```python
from build123d import *

# Parameters (mm, degrees)
SKETCH_1_W             = 800
SKETCH_1_H             = 400
EXTRUDE_1_DEPTH        = 20
SKETCH_3_W             = 302
SKETCH_3_H             = 352
CUT_EXTRUDE_1_DEPTH    = 5
CUT_EXTRUDE_2_DEPTH    = 2.7
FILLET_1_R             = 0.13
FILLET_2_R             = 0.5
FILLET_3_R             = 10
CUT_EXTRUDE_3_DEPTH    = 448.465082437
SKETCH_10_R            = 5.5
SKETCH_10_R_2          = 5
CUT_EXTRUDE_4_DEPTH    = 7
SKETCH_11_R            = 3.25
CUT_EXTRUDE_5_DEPTH    = 448.660585712
HOLE_WIZARD_M5_2_D     = 4.2
HOLE_WIZARD_M5_2_DEPTH = 14
HOLE_WIZARD_M5_2_TIP   = 1.2618073


with BuildPart() as part:
    # 스케치1 → 보스-돌출1 (new body)
    with BuildSketch(Plane(origin=(0, 0, 0), x_dir=(1, 0, 0), z_dir=(0, 1, 0))):
        Rectangle(SKETCH_1_W, SKETCH_1_H)
    extrude(amount=EXTRUDE_1_DEPTH)

    # 스케치3 → 컷-돌출1 (cut)
    with BuildSketch(Plane(origin=(0, 20, 0), x_dir=(1, 0, 0), z_dir=(0, 1, 0))):
        with Locations((200, 0)):
            Rectangle(SKETCH_3_W, SKETCH_3_H)
    extrude(amount=-CUT_EXTRUDE_1_DEPTH, mode=Mode.SUBTRACT)

    # 스케치4 → 컷-돌출2 (cut)
    with BuildSketch(Plane(origin=(0, 15, 0), x_dir=(1, 0, 0), z_dir=(0, 1, 0))):
        with BuildLine():
            Line((73.5, 168.55), (326.5, 168.55))
            ThreePointArc((326.5, 168.55), (338.556170619, 163.556170619), (343.55, 151.5))
            Line((343.55, 151.5), (343.55, -151.5))
            ThreePointArc((343.55, -151.5), (338.556170619, -163.556170619), (326.5, -168.55))
            Line((326.5, -168.55), (73.5, -168.55))
            ThreePointArc((73.5, -168.55), (61.443829381, -163.556170619), (56.45, -151.5))
            Line((56.45, -151.5), (56.45, 151.5))
            ThreePointArc((56.45, 151.5), (61.443829381, 163.556170619), (73.5, 168.55))
        make_face()
        with BuildLine():
            Line((73.5, 164.45), (326.5, 164.45))
            ThreePointArc((326.5, 164.45), (335.657032816, 160.657032816), (339.45, 151.5))
            Line((339.45, 151.5), (339.45, -151.5))
            ThreePointArc((339.45, -151.5), (335.657032816, -160.657032816), (326.5, -164.45))
            Line((326.5, -164.45), (73.5, -164.45))
            ThreePointArc((73.5, -164.45), (64.342967184, -160.657032816), (60.55, -151.5))
            Line((60.55, -151.5), (60.55, 151.5))
            ThreePointArc((60.55, 151.5), (64.342967184, 160.657032816), (73.5, 164.45))
        make_face(mode=Mode.SUBTRACT)
    extrude(amount=-CUT_EXTRUDE_2_DEPTH, mode=Mode.SUBTRACT)

    # 필렛1
    fillet_1_edges = [part.edges().sort_by_distance(p)[0] for p in [
        (61.443829381, 15, -163.556170619),
        (56.45, 15, 0),
        (61.443829381, 15, 163.556170619),
        (200, 15, 168.55),
        (338.556170619, 15, 163.556170619),
        (343.55, 15, 0),
        (338.556170619, 15, -163.556170619),
        (200, 15, -168.55),
        (64.342967184, 15, -160.657032816),
        (200, 15, -164.45),
        (335.657032816, 15, -160.657032816),
        (339.45, 15, 0),
        (335.657032816, 15, 160.657032816),
        (200, 15, 164.45),
        (64.342967184, 15, 160.657032816),
        (60.55, 15, 0),
    ]]
    fillet(fillet_1_edges, radius=FILLET_1_R)

    # 필렛2
    fillet_2_edges = [part.edges().sort_by_distance(p)[0] for p in [
        (61.443829381, 12.3, -163.556170619),
        (200, 12.3, -168.55),
        (338.556170619, 12.3, -163.556170619),
        (343.55, 12.3, 0),
        (338.556170619, 12.3, 163.556170619),
        (200, 12.3, 168.55),
        (61.443829381, 12.3, 163.556170619),
        (56.45, 12.3, 0),
        (200, 12.3, -164.45),
        (64.342967184, 12.3, -160.657032816),
        (60.55, 12.3, 0),
        (64.342967184, 12.3, 160.657032816),
        (200, 12.3, 164.45),
        (335.657032816, 12.3, 160.657032816),
        (339.45, 12.3, 0),
        (335.657032816, 12.3, -160.657032816),
    ]]
    fillet(fillet_2_edges, radius=FILLET_2_R)

    # 필렛3
    fillet_3_edges = [part.edges().sort_by_distance(p)[0] for p in [
        (351, 17.5, -176),
        (351, 17.5, 176),
        (49, 17.5, 176),
        (49, 17.5, -176),
    ]]
    fillet(fillet_3_edges, radius=FILLET_3_R)

    # 스케치6 → 컷-돌출3 (cut, through all)
    with BuildSketch(Plane(origin=(0, 15, 0), x_dir=(1, 0, 0), z_dir=(0, 1, 0))):
        with BuildLine():
            Line((80, 155), (320, 155))
            ThreePointArc((320, 155), (327.071067812, 152.071067812), (330, 145))
            Line((330, 145), (330, -145))
            ThreePointArc((330, -145), (327.071067812, -152.071067812), (320, -155))
            Line((320, -155), (80, -155))
            ThreePointArc((80, -155), (72.928932188, -152.071067812), (70, -145))
            Line((70, -145), (70, 145))
            ThreePointArc((70, 145), (72.928932188, 152.071067812), (80, 155))
        make_face()
    extrude(amount=-CUT_EXTRUDE_3_DEPTH, mode=Mode.SUBTRACT)

    # 스케치10 → 컷-돌출4 (cut)
    with BuildSketch(Plane(origin=(0, 20, 0), x_dir=(1, 0, 0), z_dir=(0, 1, 0))):
        with Locations(Location((0, 190, 0), (0, 0, 270))):
            Circle(SKETCH_10_R)
        with Locations(Location((-390, 190, 0), (0, 0, 270))):
            Circle(SKETCH_10_R)
        with Locations(Location((-390, -190, 0), (0, 0, 270))):
            Circle(SKETCH_10_R)
        with Locations(Location((0, -190, 0), (0, 0, 270))):
            Circle(SKETCH_10_R)
        with Locations(Location((390, -190, 0), (0, 0, 270))):
            Circle(SKETCH_10_R_2)
        with Locations(Location((390, 190, 0), (0, 0, 270))):
            Circle(SKETCH_10_R_2)
    extrude(amount=-CUT_EXTRUDE_4_DEPTH, mode=Mode.SUBTRACT)

    # 스케치11 → 컷-돌출5 (cut, through all)
    with BuildSketch(Plane(origin=(0, 20, 0), x_dir=(1, 0, 0), z_dir=(0, 1, 0))):
        with Locations(Location((-390, 190, 0), (0, 0, 270))):
            Circle(SKETCH_11_R)
        with Locations(Location((0, 190, 0), (0, 0, 270))):
            Circle(SKETCH_11_R)
        with Locations(Location((0, -190, 0), (0, 0, 270))):
            Circle(SKETCH_11_R)
        with Locations(Location((-390, -190, 0), (0, 0, 270))):
            Circle(SKETCH_11_R)
        with Locations(Location((390, -190, 0), (0, 0, 270))):
            Circle(SKETCH_11_R)
        with Locations(Location((390, 190, 0), (0, 0, 270))):
            Circle(SKETCH_11_R)
    extrude(amount=-CUT_EXTRUDE_5_DEPTH, mode=Mode.SUBTRACT)

    # M5 나사 구멍2
    with Locations(Plane(origin=(0, 20, 0), x_dir=(1, 0, 0), z_dir=(0, 1, 0))):
        with Locations((8.5, 120.5), (38.5, 120.5), (8.5, 60.5), (38.5, 60.5), (8.5, -60.5), (38.5, -60.5), (8.5, -120.5), (38.5, -120.5)):
            Hole(HOLE_WIZARD_M5_2_D / 2, depth=HOLE_WIZARD_M5_2_DEPTH)
            with Locations((0, 0, -(HOLE_WIZARD_M5_2_DEPTH + HOLE_WIZARD_M5_2_TIP / 2))):  # 118° drill point
                Cone(0, HOLE_WIZARD_M5_2_D / 2, HOLE_WIZARD_M5_2_TIP, mode=Mode.SUBTRACT)


solid = part.part
```
The listing builds one solid part. Answer for the finished solid, in the listing's coordinates (mm). A direction names the side the tool comes from. Give positions to 0.01 mm unless a question says otherwise; leave off trailing zeros. Order: outer loops, then holes, each group sorted by start corner. A loop starts at its lowest first (then second) coordinate and runs counter-clockwise, first axis right, second up. Notation, with made-up numbers: (15, 89.5) -> (20, 89.5) arc R21 cw to (20, 124.5) -> close; hole circle Ø2 at (67.5, 81). An arc over 180 degrees is marked (long way). Answer as a JSON object with one key per item and string values. Group by question number.
Item 1: A tool of negligible diameter and unlimited length cuts with its end or side. For faces 5 (the flat face through (-183, 20, -3)), 6 (the flat face through (202, 8, 155)), 7 (the cylindrical face through (338.42, 13.85, -163.69)), from which of +Z, -Z, +X, -X, +Y, -Y can it reach the whole face along a straight path? Write none if from no direction.
Item 2: Determine the mould class of faces 1 (the flat face through (-6, 10, -200)), 2 (the flat face through (400, 10, 3)), 3 (the flat face through (330, 8, -2)), 4 (the flat face through (-6, 10, 200)) for opening direction Z: pulls with the +Z half, pulls with the -Z half, needs draft (parallel to the pull), parting line crosses it, or undercut.
Item 3: A flat-ended cylindrical pin translates along its axis: pin 1 (10.5 mm diameter, centred on x = 0, z = -190, fed in from +Y). Find the tip coordinate at first contact, or state that the pin passes through.
Item 4: Consider L1, parallel to Z at x = 38.5, y = 14; L2, parallel to X at y = 16.75, z = -190; L3, parallel to X at y = 14.75, z = -60.5. Determine where each line is inside the solid, lowest interval first. Write a range as from..to.
Item 5: The part is cut by section A-A on z = -2.5. Write down the section's boundary in (x, y).
Result set:
{
 "1": {"face 5": "+Z, -Z, +X, -X, +Y", "face 6": "+Y, -Y", "face 7": "+Y"},
 "2": {"face 1": "pulls with the -Z half", "face 2": "needs draft", "face 3": "undercut", "face 4": "pulls with the +Z half"},
 "3": {"pin 1": "y = 13"},
 "4": {"L1": "-200..-122.6, -118.4..-62.6, -58.4..58.4, 62.6..118.4, 122.6..200", "L2": "-400..-395.5, -384.5..-5.5, 5.5..385, 395..400", "L3": "-400..6.4, 10.6..36.4, 40.6..56.45, 60.55..70, 330..339.45, 343.55..400"},
 "5": {"outline": "(-400, 0) -> (70, 0) -> (70, 15) -> (60.68, 15) arc R0.13 ccw to (60.55, 14.87) -> (60.55, 12.8) arc R0.5 cw to (60.05, 12.3) -> (56.95, 12.3) arc R0.5 cw to (56.45, 12.8) -> (56.45, 14.87) arc R0.13 ccw to (56.32, 15) -> (49, 15) -> (49, 20) -> (-400, 20) -> close; (330, 0) -> (400, 0) -> (400, 20) -> (351, 20) -> (351, 15) -> (343.68, 15) arc R0.13 ccw to (343.55, 14.87) -> (343.55, 12.8) arc R0.5 cw to (343.05, 12.3) -> (339.95, 12.3) arc R0.5 cw to (339.45, 12.8) -> (339.45, 14.87) arc R0.13 ccw to (339.32, 15) -> (330, 15) -> close"}
}
